Verification items for the finished model (mm, model axes). Give positions to 0.01 mm unless a question says otherwise; leave off trailing zeros. Loops run counter-clockwise (first coordinate to the right, second up) from the corner with the lowest first, then second, coordinate; pieces in that order, holes last. Notation, with made-up numbers: M 12,83 L 70,83 A17 cw 70,106 Z; hole C 64,22.25 d8. An arc over 180 degrees is marked long. Answer in a Markdown table with one row per item.
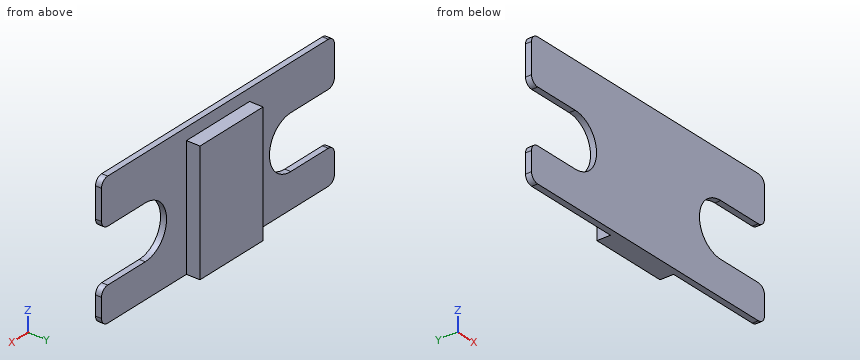
```python
from build123d import *

# Parameters (mm, degrees)
BOSS_EXTRUDE1_DEPTH = 1
FILLET1_R           = 1.27
SKETCH2_W           = 13
SKETCH2_H           = 20
BOSS_EXTRUDE2_DEPTH = 2.25


with BuildPart() as part:
    # Sketch1 → Boss-Extrude1 (new body)
    with BuildSketch(Plane(origin=(0, 0, 0), x_dir=(1, 0, 0), z_dir=(0, 1, 0))):
        with BuildLine():
            Line((0, 0), (0, 7.5))
            Line((0, 7.5), (9, 7.5))
            ThreePointArc((9, 7.5), (13.4, 11.9), (9, 16.3))
            Line((9, 16.3), (0, 16.3))
            Line((0, 16.3), (0, 22))
            Line((0, 22), (48, 22))
            Line((48, 22), (48, 16.3))
            Line((48, 16.3), (39, 16.3))
            ThreePointArc((39, 16.3), (34.6, 11.9), (39, 7.5))
            Line((39, 7.5), (48, 7.5))
            Line((48, 7.5), (48, 0))
            Line((48, 0), (0, 0))
        make_face()
    extrude(amount=BOSS_EXTRUDE1_DEPTH)

    # Fillet1
    fillet1_edges = [part.edges().sort_by_distance(p)[0] for p in [
        (0, 0.5, 0),
        (0, 0.5, -7.5),
        (0, 0.5, -16.3),
        (0, 0.5, -22),
        (48, 0.5, -22),
        (48, 0.5, -16.3),
        (48, 0.5, -7.5),
        (48, 0.5, 0),
    ]]
    fillet(fillet1_edges, radius=FILLET1_R)

    # Sketch2 → Boss-Extrude2 (add)
    with BuildSketch(Plane(origin=(0, 1, 0), x_dir=(1, 0, 0), z_dir=(0, 1, 0))):
        with Locations((24, 12)):
            Rectangle(SKETCH2_W, SKETCH2_H)
    extrude(amount=BOSS_EXTRUDE2_DEPTH)


solid = part.part
```
Item 1: Scan lines: L1, parallel to Z at x = 6, y = 0.55; L2, parallel to Y at x = 8, z = -20; L3, parallel to X at y = 2.4, z = -19.5. Record each from-to range of solid material in increasing order. Write a range as [from, to].
Reported:
| item | result |
|---|---|
| L1 | z = [-22, -16.3], [-7.5, 0] |
| L2 | y = [0, 1] |
| L3 | x = [17.5, 30.5] |
Item 2: Sectioned sample at A-A (x = 5.5). Record the cut outline in (y, z).
Reported:
| item | result |
|---|---|
| outline | M 0,-22 L 1,-22 L 1,-16.3 L 0,-16.3 Z; M 0,-7.5 L 1,-7.5 L 1,0 L 0,0 Z |
Item 3: Go/stop test with flat-tipped pins: pin 1 (4 mm diameter, centred on x = 43, z = -6, fed in from +Y); pin 2 (1.8 mm diameter, centred on y = 2, z = -16, fed in from +X); pin 3 (0.7 mm diameter, centred on y = 2, z = -13, fed in from -X). Record where each tip stops, or that it passes through.
Reported:
| item | result |
|---|---|
| pin 1 | stops at y = 1 |
| pin 2 | stops at x = 30.5 |
| pin 3 | stops at x = 17.5 |
Item 4: Sectioned sample at B-B (z = -5.75). Record the cut outline in (x, y).
Reported:
| item | result |
|---|---|
| outline | M 0,0 L 48,0 L 48,1 L 30.5,1 L 30.5,3.25 L 17.5,3.25 L 17.5,1 L 0,1 Z |
Item 5: Sectioned sample at C-C (y = 0.55). Record the cut outline in (x, z), and give its area (3 significant figures).
Reported:
| item | result |
|---|---|
| outline | M 0,-20.73 A1.27 ccw 1.27,-22 L 46.73,-22 A1.27 ccw 48,-20.73 L 48,-17.57 A1.27 ccw 46.73,-16.3 L 39,-16.3 A4.4 cw 39,-7.5 L 46.73,-7.5 A1.27 ccw 48,-6.23 L 48,-1.27 A1.27 ccw 46.73,0 L 1.27,0 A1.27 ccw 0,-1.27 L 0,-6.23 A1.27 ccw 1.27,-7.5 L 9,-7.5 A4.4 cw 9,-16.3 L 1.27,-16.3 A1.27 ccw 0,-17.57 Z |
| area | 834 mm^2 |
Item 6: Sectioned sample at D-D (x = 27.5). Record the cut outline in (y, z).
Reported:
| item | result |
|---|---|
| outline | M 0,-22 L 3.25,-22 L 3.25,-2 L 1,-2 L 1,0 L 0,0 Z |
